Part model, mm, in its own coordinate system. Face numbers are marked on the shaded views. A direction names the side the tool comes from. Give positions to 0.01 mm unless a question says otherwise; leave off trailing zeros. Write each loop counter-clockwise with the first axis right and the second up, starting at its lowest first coordinate (ties: lowest second). Pieces come first, ordered by that corner, then holes. Notation, with made-up numbers: M -5,-20 L 36,-20 A17 ccw 36,-1 Z; hole C 6.25,31 d4. An arc over 180 degrees is marked long. Use a Markdown table: item, result. Add a question column.
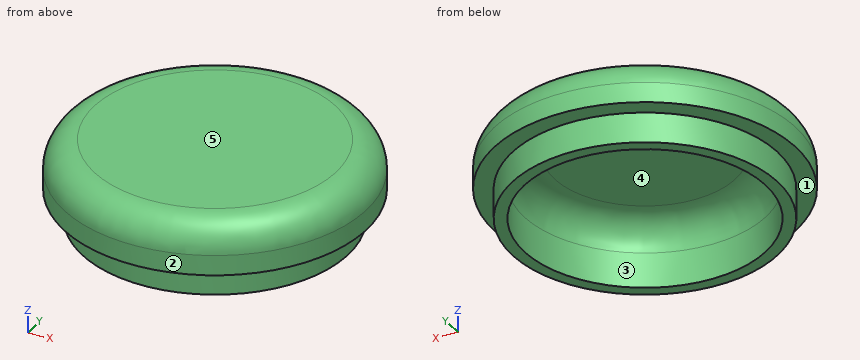
from build123d import *

# Parameters (mm, degrees)
SKETCH1_R           = 15
BOSS_EXTRUDE1_DEPTH = 5
FILLET1_R           = 3
SKETCH2_R           = 12
CUT_EXTRUDE1_DEPTH  = 3.5
FILLET2_R           = 3
SKETCH4_R           = 13.2
BOSS_EXTRUDE3_DEPTH = 3
SKETCH5_R           = 12
CUT_EXTRUDE2_DEPTH  = 3


with BuildPart() as part:
    # Sketch1 → Boss-Extrude1 (new body)
    with BuildSketch(Plane.XY):
        Circle(SKETCH1_R)
    extrude(amount=BOSS_EXTRUDE1_DEPTH)

    # Fillet1
    fillet1_edges = [part.edges().sort_by_distance(p)[0] for p in [
        (-15, 0, 5),
    ]]
    fillet(fillet1_edges, radius=FILLET1_R)

    # Sketch2 → Cut-Extrude1 (cut)
    with BuildSketch(Plane(origin=(0, 0, 0), x_dir=(-1, 0, 0), z_dir=(0, 0, -1))):
        Circle(SKETCH2_R)
    extrude(amount=-CUT_EXTRUDE1_DEPTH, mode=Mode.SUBTRACT)

    # Fillet2
    fillet2_edges = [part.edges().sort_by_distance(p)[0] for p in [
        (12, 0, 3.5),
    ]]
    fillet(fillet2_edges, radius=FILLET2_R)

    # Sketch4 → Boss-Extrude3 (add)
    with BuildSketch(Plane(origin=(0, 0, 0), x_dir=(-1, 0, 0), z_dir=(0, 0, -1))):
        Circle(SKETCH4_R)
    extrude(amount=BOSS_EXTRUDE3_DEPTH)

    # Sketch5 → Cut-Extrude2 (cut)
    with BuildSketch(Plane(origin=(0, 0, -3), x_dir=(-1, 0, 0), z_dir=(0, 0, -1))):
        Circle(SKETCH5_R)
    extrude(amount=-CUT_EXTRUDE2_DEPTH, mode=Mode.SUBTRACT)


solid = part.part
1. Cut at C-C (z = -1). Write the cut outline in (x, y).
2. Cut at A-A (y = 0). Write the cut outline in (x, z).
3. Flat gauge pins, fed straight in: pin 1 (1 mm diameter, centred on x = 8, z = 0.5, fed in from +Y); pin 2 (6 mm diameter, centred on x = 4.5, y = -0.5, fed in from -Z); pin 3 (1.5 mm diameter, centred on y = -5.5, z = -2, fed in from -X). Where does each tip first touch, or does it go through?
4. Mould opens along Y. For the marked faces 1, 2 and 3 say: released by +Y, released by -Y, zero draft, split by the parting line, or undercut.
5. Cut at D-D (z = 3). Write the cut outline in (x, y), then the cut area to 3 significant figures.
6. Tool access for the marked faces 4 and 5: list every direction of +Z, -Z, +X, -X, +Y, -Y with a clear straight run to the whole face (end or side of a thin tool).
7. Drill centre lines: probe 1 along Y at (x, z) = (0, -0.4); probe 2 along Z at (x, y) = (6, 1); probe 3 along X at (y, z) = (6.25, -1). Where is each one in solid material? Low to high. Write a range as [from, to].
A:
| question | item | result |
|---|---|---|
| 1 | outline | C 0,0 d26.4; hole C 0,0 d24 |
| 2 | outline | M -15,0 L -13.2,0 L -13.2,-3 L -12,-3 L -12,0.5 A3 cw -9,3.5 L 9,3.5 A3 cw 12,0.5 L 12,-3 L 13.2,-3 L 13.2,0 L 15,0 L 15,2 A3 ccw 12,5 L -12,5 A3 ccw -15,2 Z |
| 3 | pin 1 | stops at y = 12.99 |
| 3 | pin 2 | stops at z = 3.5 |
| 3 | pin 3 | stops at x = -12.32 |
| 4 | face 1 | zero draft |
| 4 | face 2 | split by the parting line |
| 4 | face 3 | undercut |
| 5 | outline | C 0,0 d29.66; hole C 0,0 d21.32 |
| 5 | area | 334 mm² |
| 6 | face 4 | -Z |
| 6 | face 5 | +Z, +X, -X, +Y, -Y |
| 7 | probe 1 | y = [-13.2, -12], [12, 13.2] |
| 7 | probe 2 | z = [3.5, 5] |
| 7 | probe 3 | x = [-11.63, -10.24], [10.24, 11.63] |
